Model file for the job. Use its own axes, mm. A direction names the side the tool comes from. Give positions to 0.01 mm unless a question says otherwise; leave off trailing zeros. Loops run counter-clockwise (first coordinate to the right, second up) from the corner with the lowest first, then second, coordinate; pieces in that order, holes last. Notation, with made-up numbers: M -32,57.25 L 6,57.25 A12 ccw 6,79.25 Z; hole C 11,67.25 d8. An arc over 180 degrees is marked long. Answer in a Markdown table with one row per item.
```python
from build123d import *

# Parameters (mm, degrees)
SKETCH9_W           = 21.65
SKETCH9_H           = 6.35
SKETCH9_W_2         = 6.35
SKETCH9_H_2         = 51.65
BOSS_EXTRUDE1_DEPTH = 6.35
FILLET2_R           = 5
FILLET3_R           = 7


with BuildPart() as part:
    # Sketch9 → Boss-Extrude1 (new body)
    with BuildSketch(Plane(origin=(0, 0, 0), x_dir=(1, 0, 0), z_dir=(0, 1, 0))):
        with Locations((10.825, -3.175)):
            Rectangle(SKETCH9_W, SKETCH9_H)
        with Locations((24.825, -3.175)):
            Rectangle(SKETCH9_W_2, SKETCH9_H)
        with Locations((24.825, -32.175)):
            Rectangle(SKETCH9_W_2, SKETCH9_H_2)
    extrude(amount=BOSS_EXTRUDE1_DEPTH)

    # Fillet2
    fillet2_edges = [part.edges().sort_by_distance(p)[0] for p in [
        (21.65, 3.175, 6.35),
    ]]
    fillet(fillet2_edges, radius=FILLET2_R)

    # Fillet3
    fillet3_edges = [part.edges().sort_by_distance(p)[0] for p in [
        (28, 3.175, 0),
    ]]
    fillet(fillet3_edges, radius=FILLET3_R)


solid = part.part
```
Q1. Saw through at C-C (z = 14). Give the cut face in (x, y).
Reported:
| item | result |
|---|---|
| outline | M 21.65,0 L 28,0 L 28,6.35 L 21.65,6.35 Z |
Q2. 3-axis set-ups, long thin cutter, end or side, ignore diameter. For faces 1 (the face through (28, 3, 33)), 2 (the face through (8, 3, 6.35)): which of +Z, -Z, +X, -X, +Y, -Y reach the whole face in a straight line?
Reported:
| item | result |
|---|---|
| face 1 | +Z, -Z, +X, +Y, -Y |
| face 2 | +Z, -X, +Y, -Y |
Q3. Saw through at B-B (x = 3.75). Give the cut face in (y, z).
Reported:
| item | result |
|---|---|
| outline | M 0,0 L 6.35,0 L 6.35,6.35 L 0,6.35 Z |
Q4. Saw through at A-A (y = 3). Give the cut face in (x, z), and give its area (3 significant figures).
Reported:
| item | result |
|---|---|
| outline | M 0,0 L 21,0 A7 ccw 28,7 L 28,58 L 21.65,58 L 21.65,11.35 A5 cw 16.65,6.35 L 0,6.35 Z |
| area | 501 mm² |
Q5. Drop flat-ended pins along their axis: pin 1 (1.9 mm diameter, centred on x = 6, y = 3.5, fed in from +Z); pin 2 (3 mm diameter, centred on y = 4, z = 43, fed in from -X). Give the stop position or say it passes through.
Reported:
| item | result |
|---|---|
| pin 1 | z = 6.35 |
| pin 2 | x = 21.65 |
Q6. Probe probe 1 along X at (y, z) = (1.75, 33); probe 2 along Z at (x, y) = (12.5, 4.5); probe 3 along X at (y, z) = (3.25, 5.5). List the from-to ranges inside material, lowest first.
Reported:
| item | result |
|---|---|
| probe 1 | 21.65 to 28 |
| probe 2 | 0 to 6.35 |
| probe 3 | 0 to 27.84 |
